from build123d import *

# Parameters (mm, degrees)
F0_W     = 101.6
F0_H     = 63.5
F1_DEPTH = 9.398
F3_D     = 12.6238
F4_D     = 14.6812
F5_R     = 2.54
F6_D     = 4.0386


with BuildPart() as f1:
    # F0 (on Front) → F1 (new body)
    with BuildSketch(Plane.XZ):
        Rectangle(F0_W, F0_H)
    extrude(amount=F1_DEPTH)

    # F3 (through all)
    with Locations(Plane.XZ.offset(9.398)):
        with Locations((-38.1, 19.05)):
            Hole(F3_D / 2)

    # F4 (through all)
    with Locations(Plane.XZ.offset(9.398)):
        with Locations((38.1, 19.05)):
            Hole(F4_D / 2)

    # F5
    f5_edges = [f1.edges().sort_by_distance(p)[0] for p in [
        (0, -9.398, 31.75),
        (-50.8, -9.398, 0),
        (50.8, -9.398, 0),
        (0, -9.398, -31.75),
        (50.8, 0, 0),
        (-50.8, 0, 0),
        (0, 0, -31.75),
        (0, 0, 31.75),
    ]]
    fillet(f5_edges, radius=F5_R)

    # F6 (through all)
    with Locations(Plane.XZ.offset(9.398)):
        with Locations((0, 19.05)):
            Hole(F6_D / 2)


solid = f1.part
The listing builds one solid part. Answer for the finished solid, in the listing's coordinates (mm). Coordinates: 2 decimals unless noted, no trailing zeros. Write each loop counter-clockwise with the first axis right and the second up, starting at its lowest first coordinate (ties: lowest second). Pieces come first, ordered by that corner, then holes. Notation, with made-up numbers: (-5.75, -31) - (-0.75, -31) arc R20 cw to (-0.75, 5) - close; hole circle Ø11 at (66.25, 27.25). An arc over 180 degrees is marked (long way). Put each result on its own line as item: value.
1. The part is cut by section C-C on z = 19.05. Give the vertices of the cut face in (x, y).
Answer sheet:
outline: (-50.8, -6.86) arc R2.54 ccw to (-48.26, -9.4) - (-44.41, -9.4) - (-44.41, 0) - (-48.26, 0) arc R2.54 ccw to (-50.8, -2.54) - close; (-31.79, -9.4) - (-2.02, -9.4) - (-2.02, 0) - (-31.79, 0) - close; (2.02, -9.4) - (30.76, -9.4) - (30.76, 0) - (2.02, 0) - close; (45.44, -9.4) - (48.26, -9.4) arc R2.54 ccw to (50.8, -6.86) - (50.8, -2.54) arc R2.54 ccw to (48.26, 0) - (45.44, 0) - close
2. The part is cut by section D-D on x = -38.1. Give the vertices of the cut face in (y, z).
Answer sheet:
outline: (-9.4, -29.21) arc R2.54 ccw to (-6.86, -31.75) - (-2.54, -31.75) arc R2.54 ccw to (0, -29.21) - (0, 12.74) - (-9.4, 12.74) - close; (-9.4, 25.36) - (0, 25.36) - (0, 29.21) arc R2.54 ccw to (-2.54, 31.75) - (-6.86, 31.75) arc R2.54 ccw to (-9.4, 29.21) - close
3. The part is cut by section B-B on y = -5.75. Give the vertices of the cut face in (x, z), plus the area to 3 significant figures.
Answer sheet:
outline: (-50.8, -31.75) - (50.8, -31.75) - (50.8, 31.75) - (-50.8, 31.75) - close; hole circle Ø12.62 at (-38.1, 19.05); hole circle Ø4.04 at (0, 19.05); hole circle Ø14.68 at (38.1, 19.05)
area: 6,140 mm^2
4. Determine the mould class of faces 1 (the face through (50.04, -8.67, 0.44)), 2 (the face through (31.32, -4.63, 16.24)), 3 (the face through (0.711, -0.764, 31.026)) for opening direction Z: pulls with the +Z half, pulls with the -Z half, needs draft (parallel to the pull), parting line crosses it, or undercut.
Answer sheet:
face 1: needs draft
face 2: undercut
face 3: pulls with the +Z half
5. The part is cut by section A-A on x = 38.1. Give the vertices of the cut face in (y, z), plus the area to 3 significant figures.
Answer sheet:
outline: (-9.4, -29.21) arc R2.54 ccw to (-6.86, -31.75) - (-2.54, -31.75) arc R2.54 ccw to (0, -29.21) - (0, 11.71) - (-9.4, 11.71) - close; (-9.4, 26.39) - (0, 26.39) - (0, 29.21) arc R2.54 ccw to (-2.54, 31.75) - (-6.86, 31.75) arc R2.54 ccw to (-9.4, 29.21) - close
area: 453 mm^2
6. Find the intervals of material crossed by line 1 along X through (y, z) = (-7.25, 14.5); line 2 along Z through (x, y) = (-38.1, -6), in increasing order. Write a range as from..to.
Answer sheet:
line 1: x = -50.77..-42.47, -33.73..32.34, 43.86..50.77
line 2: z = -31.75..12.74, 25.36..31.75
